Check sheet for the modelled part. Datum: model origin and axes. Units: mm. A direction names the side the tool comes from. Round coordinates to 2 decimals unless told otherwise and drop trailing zeros. Write each loop counter-clockwise with the first axis right and the second up, starting at its lowest first coordinate (ties: lowest second). Pieces come first, ordered by that corner, then holes.
from build123d import *

# Parameters (mm, degrees)
CROQUIS1_R              = 33.485
SALIENTE_EXTRUIR1_DEPTH = 2
CROQUIS2_R              = 35.775
SALIENTE_EXTRUIR2_DEPTH = 6.52
SALIENTE_EXTRUIR3_START = 37
CROQUIS3_R              = 33.485
SALIENTE_EXTRUIR3_DEPTH = 37
CROQUIS4_R              = 9.04
SALIENTE_EXTRUIR4_DEPTH = 2
CROQUIS5_R              = 2.425
SALIENTE_EXTRUIR5_DEPTH = 0.5
CROQUIS6_R              = 0.5
CORTAR_EXTRUIR1_DEPTH   = 1
CROQUIS7_R              = 3
SALIENTE_EXTRUIR6_DEPTH = 36
REDONDEO2_R             = 2


with BuildPart() as part:
    # Croquis1 → Saliente-Extruir1 (new, symmetric)
    with BuildSketch(Plane.XY):
        Circle(CROQUIS1_R)
    extrude(amount=SALIENTE_EXTRUIR1_DEPTH, both=True)

    # Croquis2 → Saliente-Extruir2 (add)
    with BuildSketch(Plane.XY.offset(2)):
        Circle(CROQUIS2_R)
    extrude(amount=SALIENTE_EXTRUIR2_DEPTH)

    # Croquis3 → Saliente-Extruir3 (add)
    with BuildSketch(Plane.XY.offset(8.52).offset(SALIENTE_EXTRUIR3_START)):
        Circle(CROQUIS3_R)
    extrude(amount=-SALIENTE_EXTRUIR3_DEPTH)

    # Croquis4 → Saliente-Extruir4 (add)
    with BuildSketch(Plane.XY.offset(45.52)):
        Circle(CROQUIS4_R)
    extrude(amount=SALIENTE_EXTRUIR4_DEPTH)

    # Croquis5 → Saliente-Extruir5 (add)
    with BuildSketch(Plane.XY.offset(47.52)):
        Circle(CROQUIS5_R)
    extrude(amount=SALIENTE_EXTRUIR5_DEPTH)

    # Croquis6 → Cortar-Extruir1 (cut)
    with BuildSketch(Plane.XY.offset(48.02)):
        Circle(CROQUIS6_R)
    extrude(amount=-CORTAR_EXTRUIR1_DEPTH, mode=Mode.SUBTRACT)

    # Croquis7 → Saliente-Extruir6 (add)
    with BuildSketch(Plane(origin=(0, 0, -2), x_dir=(-1, 0, 0), z_dir=(0, 0, -1))):
        with Locations(Location((0, 0, 0), (0, 0, 180))):
            Circle(CROQUIS7_R)
    extrude(amount=SALIENTE_EXTRUIR6_DEPTH)

    # Redondeo2
    redondeo2_edges = [part.edges().sort_by_distance(p)[0] for p in [
        (-33.485, 0, 45.52),
    ]]
    fillet(redondeo2_edges, radius=REDONDEO2_R)


solid = part.part
1. Scan lines: line 1 along Z through (x, y) = (-4, -1); line 2 along Z through (x, y) = (25, 3.5); line 3 along X through (y, z) = (-19.5, 7.5). Record each from-to range of solid material in increasing order.
2. Go/stop test with flat-tipped pins: pin 1 (12 mm diameter, centred on x = 7.5, z = 9, fed in from -Y); pin 2 (4 mm diameter, centred on y = 6, z = 3, fed in from -X); pin 3 (8 mm diameter, centred on y = 4, z = -19, fed in from +X). Record where each tip stops, or that it passes through.
3. Set-up check for faces 1 (the cylindrical face through (-1.96, -8.825, 46.506)), 2 (the cylindrical face through (2.86, -0.9, -19.75)), 3 (the flat face through (1, 0, 48.02)): record each of +Z, -Z, +X, -X, +Y, -Y from which the full face is reachable in a straight line by a thin tool's end or side.
4. Sectioned sample at A-A, the plane z = 15. Enter the section's corners in (x, y) (3 decimals), plus the area to 3 significant figures.
Computed values:
1. line 1: z = -2 to 47.52
1. line 2: z = -2 to 45.52
1. line 3: x = -29.99 to 29.99
2. pin 1: stops at y = -35.74
2. pin 2: stops at x = -35.55
2. pin 3: stops at x = 3
3. face 1: +Z
3. face 2: -Z
3. face 3: +Z, +X, -X, +Y, -Y
4. outline: circle Ø66.97 at (0, 0)
4. area: 3,520 mm2
